Here's how the part is built. I have some questions about the finished solid (model axes, mm). Face numbers are marked on the shaded views. A direction names the side the tool comes from. Give positions to 0.01 mm unless a question says otherwise; leave off trailing zeros. Order: outer loops, then holes, each group sorted by start corner. A loop starts at its lowest first (then second) coordinate and runs counter-clockwise, first axis right, second up. Notation, with made-up numbers: M -40,-36.5 L -7,-36.5 A25 cw -7,-2.5 Z; hole C 14,-28.75 d5. An arc over 180 degrees is marked long. Use one line per item in the form item = value.
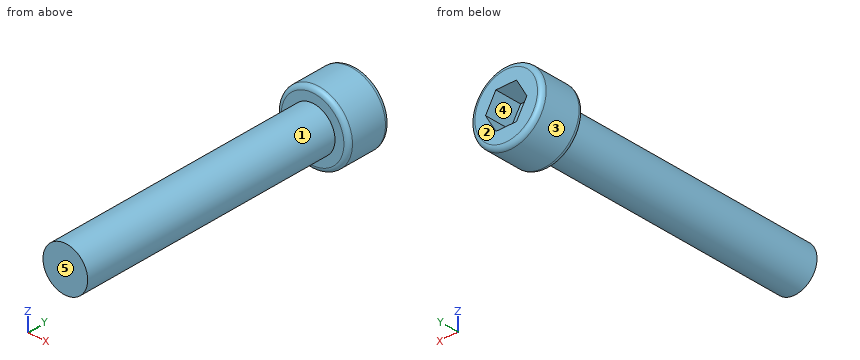
from build123d import *

# Parameters (mm, degrees)
F0_R     = 2.5
F1_DEPTH = 30
F2_R     = 4
F3_DEPTH = 5
F4_R     = 0.5
F6_DEPTH = 3


with BuildPart() as f1:
    # F0 (on Front) → F1 (new body)
    with BuildSketch(Plane.XZ):
        Circle(F0_R)
    extrude(amount=-F1_DEPTH)

    # F2 (on face) → F3 (join)
    with BuildSketch(Plane(origin=(0, 30, 0), x_dir=(-1, 0, 0), z_dir=(0, 1, 0))):
        Circle(F2_R)
    extrude(amount=F3_DEPTH)

    # F4
    f4_edges = [f1.edges().sort_by_distance(p)[0] for p in [
        (4, 30, 0),
        (4, 35, 0),
    ]]
    fillet(f4_edges, radius=F4_R)

    # F5 (on face) → F6 (cut)
    with BuildSketch(Plane(origin=(0, 35, 0), x_dir=(-1, 0, 0), z_dir=(0, 1, 0))):
        Polygon((1.154701, 2), (-1.154701, 2), (-2.309401, 0), (-1.154701, -2), (1.154701, -2), (2.309401, 0), align=None)
    extrude(amount=-F6_DEPTH, mode=Mode.SUBTRACT)


solid = f1.part
Q1. I'm going to push flat-ended pins straight in: pin 1 Ø2 at (x, y) = (0, 26) entering from -Z; pin 2 Ø2 at (x, y) = (-2, 7) entering from -Z; pin 3 Ø0.7 at (x, y) = (0.5, 33) entering from -Z. Where does each tip first touch, or does it pass through?
Found:
pin_1 = -2.5
pin_2 = -2.29
pin_3 = -4
Q2. On a 3-axis mill with a long thin cutter (end or side, diameter ignored), from which of +Z, -Z, +X, -X, +Y, -Y can I reach the whole of each face in a straight line? I mean the marked faces 1 and 2. Say none if no direction works.
Found:
face_1 = -Y
face_2 = +Z, -Z, +X, -X, +Y
Q3. I want a section at B-B on y = 25. Write out the boundary of the cut face in (x, z).
Found:
outline = C 0,0 d5
Q4. Thinking about a two-plate mould opening in X: for the marked faces 3, 4 and 5, which applies, +X half, -X half, draft (parallel to the pull), parting line (faces both ways), or undercut?
Found:
face_3 = parting line
face_4 = undercut
face_5 = draft
Q5. I want a section at A-A on x = 0. Write out the boundary of the cut face in (y, z), then the cut area to 3 significant figures.
Found:
outline = M 0,-2.5 L 30,-2.5 L 30,-3.5 A0.5 ccw 30.5,-4 L 34.5,-4 A0.5 ccw 35,-3.5 L 35,-2 L 32,-2 L 32,2 L 35,2 L 35,3.5 A0.5 ccw 34.5,4 L 30.5,4 A0.5 ccw 30,3.5 L 30,2.5 L 0,2.5 Z
area = 178 mm²
Q6. I need wall thicknesses on L1, parallel to Y at x = 2.25, z = 2.5; L2, parallel to Z at x = 0, y = 9; L3, parallel to Y at x = -0.25, z = -0.25. Which ranges of each line are inside material? Lowest first, please.
Found:
L1 = 30 to 35
L2 = -2.5 to 2.5
L3 = 0 to 32
